```python
from build123d import *

# Parameters (mm, degrees)
BOSS_EXTRUDE1_DEPTH = 1.2
SKETCH2_R           = 1.6
CUT_EXTRUDE1_DEPTH  = 1.2
SKETCH3_W           = 2.2
SKETCH3_H           = 2.2
BOSS_EXTRUDE2_DEPTH = 1.6


with BuildPart() as part:
    # Sketch1 → Boss-Extrude1 (new body)
    with BuildSketch(Plane(origin=(0, 0, 0), x_dir=(1, 0, 0), z_dir=(0, 1, 0))):
        Polygon((87.2, 5.6), (72, 5.6), (0, 0), (-14, 0), (-14, -16), (0, -16), (87.2, -10.6), align=None)
    extrude(amount=BOSS_EXTRUDE1_DEPTH)

    # Sketch2 → Cut-Extrude1 (cut)
    with BuildSketch(Plane(origin=(0, 1.2, 0), x_dir=(1, 0, 0), z_dir=(0, 1, 0))):
        with Locations((-6, -12)):
            Circle(SKETCH2_R)
        with Locations((83.6, 2)):
            Circle(SKETCH2_R)
    extrude(amount=-CUT_EXTRUDE1_DEPTH, mode=Mode.SUBTRACT)

    # Sketch3 → Boss-Extrude2 (add)
    with BuildSketch(Plane(origin=(0, 1.2, 0), x_dir=(1, 0, 0), z_dir=(0, 1, 0))):
        with Locations((-6.5, -7.6)):
            Rectangle(SKETCH3_W, SKETCH3_H)
    extrude(amount=BOSS_EXTRUDE2_DEPTH)


solid = part.part
```
The listing builds one solid part. Answer for the finished solid, in the listing's coordinates (mm). A direction names the side the tool comes from. Round coordinates to 2 decimals unless told otherwise and drop trailing zeros. Write each loop counter-clockwise with the first axis right and the second up, starting at its lowest first coordinate (ties: lowest second). Pieces come first, ordered by that corner, then holes. Notation, with made-up numbers: (75, 56) -> (112, 56) arc R20 ccw to (112, 72) -> close; hole circle Ø5 at (35.25, -34). An arc over 180 degrees is marked (long way). Write item = value, one per line.
1) Given pin 1 (2 mm diameter, centred on x = 34.5, z = 12.5, fed in from +Y); pin 2 (10 mm diameter, centred on x = 33, z = 7, fed in from -Y); pin 3 (1 mm diameter, centred on x = -10, y = 0.5, fed in from -Z); pin 4 (1.3 mm diameter, centred on x = -7, y = 2, fed in from -Z), each flat-ended and moving along its own axis, determine where each tip first touches the part or whether it passes through.
Check values:
pin_1 = 1.2
pin_2 = 0
pin_3 = 0
pin_4 = 6.5
2) Which of the six approach directions +Z, -Z, +X, -X, +Y, -Y give full straight-line access (tool end or side, diameter ignored) to faces 1 (the flat face through (-7, 2, 6.5)), 2 (the flat face through (-7, 2, 8.7)), 3 (the flat face through (-5.4, 2, 8)), 4 (the flat face through (-7.6, 2, 8))?
Check values:
face_1 = -Z, +X, -X, +Y
face_2 = +Z, +X, -X, +Y
face_3 = +Z, -Z, +X, +Y
face_4 = +Z, -Z, -X, +Y
3) Straight lines are drawn through the part: line 1 along Z through (x, y) = (-6, 0.3); line 2 along Y through (x, z) = (43, 1.25); line 3 along Z through (x, y) = (83.6, 0.45). For each, find the intervals that lie inside material, in ascending order. Write a range as [from, to].
Check values:
line_1 = [0, 10.4], [13.6, 16]
line_2 = [0, 1.2]
line_3 = [-5.6, -3.6], [-0.4, 10.82]
4) Section B-B on x = 83.6 is taken. Write down the section's boundary in (y, z), plus the area to 3 significant figures.
Check values:
outline = (0, -5.6) -> (1.2, -5.6) -> (1.2, -3.6) -> (0, -3.6) -> close; (0, -0.4) -> (1.2, -0.4) -> (1.2, 10.82) -> (0, 10.82) -> close
area = 15.9 mm²
5) Section C-C on z = -2 is taken. Write down the section's boundary in (x, y).
Check values:
outline = (25.71, 0) -> (82, 0) -> (82, 1.2) -> (25.71, 1.2) -> close; (85.2, 0) -> (87.2, 0) -> (87.2, 1.2) -> (85.2, 1.2) -> close
6) Section A-A on y = 0.5 is taken. Write down the section's boundary in (x, z), plus the area to 3 significant figures.
Check values:
outline = (-14, 0) -> (0, 0) -> (72, -5.6) -> (87.2, -5.6) -> (87.2, 10.6) -> (0, 16) -> (-14, 16) -> close; hole circle Ø3.2 at (-6, 12); hole circle Ø3.2 at (83.6, -2)
area = 1,650 mm²
7) Section D-D on x = 10 is taken. Write down the section's boundary in (y, z).
Check values:
outline = (0, -0.78) -> (1.2, -0.78) -> (1.2, 15.38) -> (0, 15.38) -> close
8) For a pull along Z with two mould halves and no side action, classify faces 5 (the cylindrical face through (85.126, 0.608, -2.481)), 6 (the flat face through (42.99, 0.592, 13.338)), 7 (the cylindrical face through (-5.26, 0.61, 13.42)), 8 (the flat face through (36, 1.2, 5)) as released by +Z, released by -Z, zero draft, split by the parting line, or undercut.
Check values:
face_5 = undercut
face_6 = released by +Z
face_7 = undercut
face_8 = zero draft
